For this review, use the dimensioned drawing (mm, ordinates from the lowest corner) and the shaded views. A direction names the side the tool comes from. Coordinates: 2 decimals unless noted, no trailing zeros. Write each loop counter-clockwise with the first axis right and the second up, starting at its lowest first coordinate (ties: lowest second). Pieces come first, ordered by that corner, then holes. Notation, with made-up numbers: (-20, 31) - (-7, 31) arc R17 cw to (-7, 49) - close; hole circle Ø2 at (73.5, 37). An arc over 180 degrees is marked (long way). Use one line per item in the form item = value. Start each with the question number.
1) Tool access review of the marked faces 1, 2, 3 and 4: name each direction out of +Z, -Z, +X, -X, +Y, -Y from which nothing blocks a thin tool from reaching the whole face with its end or side.
2) Insertion check: P1, Ø1, axis at x = 13, y = 11, coming from the +Z side; P2, Ø3, axis at y = 10, z = 42, coming from the -X side (3 decimals); P3, Ø4, axis at x = 9, z = 18, coming from the +Y side. Each pin has a flat end and moves straight along its axis. Give the tip position at first contact, or say it passes through.
3) For L1, parallel to Z at x = 4.25, y = 4.25; L2, parallel to Y at x = 5.75, z = 20 (1 decimal); L3, parallel to Y at x = 7.25, z = 8 (1 decimal), list the stretches that pass through material, from the lowest coordinate up. Write a range as from..to.
4) We need section A-A (z = 5). Give the boundary of the cut face in (x, y).
5) We need section B-B (y = 8). Give the boundary of the cut face in (x, z), plus the area to 3 significant figures.
6) We need section D-D (z = 25.5). Give the boundary of the cut face in (x, y).
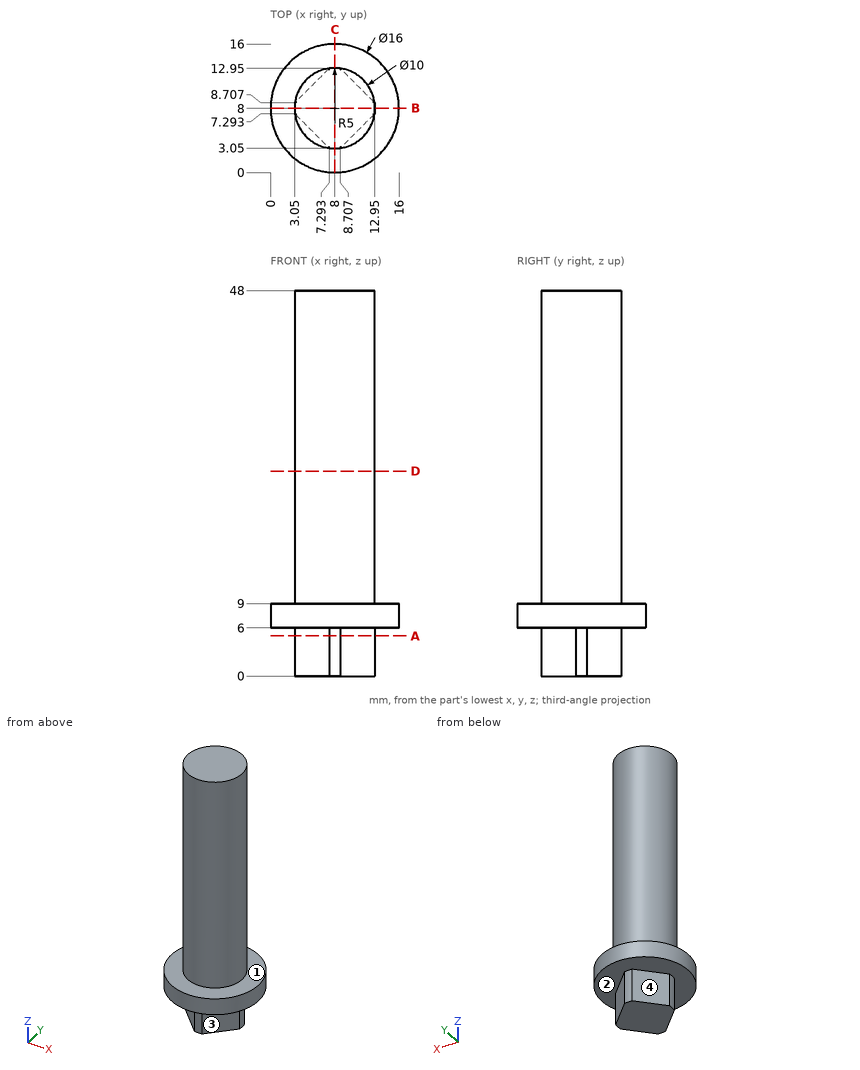
Determined:
q1.face_1 = +Z
q1.face_2 = -Z
q1.face_3 = -Z, +X, -Y
q1.face_4 = -Z, -X, +Y
q2.P1 = 9
q2.P2 = 3.025
q2.P3 = 13
q3.L1 = 6..9
q3.L2 = 3.5..12.5
q3.L3 = 0..16
q4.outline = (3.05, 7.29) - (7.29, 3.05) arc R5 ccw to (8.71, 3.05) - (12.95, 7.29) arc R5 ccw to (12.95, 8.71) - (8.71, 12.95) arc R5 ccw to (7.29, 12.95) - (3.05, 8.71) arc R5 ccw to start
q5.outline = (0, 6) - (3, 6) - (3, 0) - (13, 0) - (13, 6) - (16, 6) - (16, 9) - (13, 9) - (13, 48) - (3, 48) - (3, 9) - (0, 9) - close
q5.area = 498 mm²
q6.outline = circle Ø10 at (8, 8)
